```python
from build123d import *

# Parameters (mm, degrees)
EXTRUDE_275_DEPTH = 17
SKETCH_2_R        = 12.9
EXTRUDE_1_DEPTH   = 200
FILLET_3_R        = 2
SKETCH_3_R        = 11
EXTRUDE_2_DEPTH   = 100
FILLET_4_R        = 2


with BuildPart() as part:
    # 草图1 → Extrude 275 (new body)
    with BuildSketch(Plane.XY):
        Polygon((20.984201837, 10.954296262), (1.005402075, 23.65), (-19.978799762, 12.695703738), (-20.984201837, -10.954296262), (-1.005402075, -23.65), (19.978799762, -12.695703738), align=None)
    extrude(amount=EXTRUDE_275_DEPTH)

    # 草图2 → 凸台-拉伸1 (add)
    with BuildSketch(Plane.XY.offset(17)):
        with Locations(Location((0, 0, 0), (0, 0, 180))):
            Circle(SKETCH_2_R)
    extrude(amount=EXTRUDE_1_DEPTH)

    # 圆角3
    fillet_3_edges = [part.edges().sort_by_distance(p)[0] for p in [
        (9.486698843, -18.172851869, 0),
        (-10.994801956, -17.302148131, 0),
        (-20.4815008, 0.870703738, 0),
        (-9.486698843, 18.172851869, 0),
        (10.994801956, 17.302148131, 0),
        (20.4815008, -0.870703738, 0),
    ]]
    fillet(fillet_3_edges, radius=FILLET_3_R)

    # 草图3 → 凸台-拉伸2 (add)
    with BuildSketch(Plane.XY.offset(217)):
        Circle(SKETCH_3_R)
    extrude(amount=EXTRUDE_2_DEPTH)

    # 圆角4
    fillet_4_edges = [part.edges().sort_by_distance(p)[0] for p in [
        (-11, 0, 317),
    ]]
    fillet(fillet_4_edges, radius=FILLET_4_R)


solid = part.part
```
Source: CAD feature listing. Evaluate the final solid. Frame: model axes, mm. A direction names the side the tool comes from. Coordinates: 2 decimals unless noted, no trailing zeros. Order: outer loops, then holes, each group sorted by start corner. A loop starts at its lowest first (then second) coordinate and runs counter-clockwise, first axis right, second up. Notation, with made-up numbers: M 2.25,51 L 58.25,51 A34 cw 58.25,83 Z; hole C 89,-32 d6. An arc over 180 degrees is marked long. Write each question's results on one line, items separated by ' | '. Start each with the question number.
1) Access query for faces 1 (the face through (-11.135, -17.213, 9.395)), 2 (the face through (9, -10, 17)). Directions: +Z, -Z, +X, -X, +Y, -Y. A direction counts if a zero-diameter tool reaches every point of the face in a straight line with its end or side. Return the directions, or none.
2) Section query A-A (z = 85). Return the cut outline in (x, y).
3) Line query: line 1 (X direction, y = 2, z = 62); line 2 (Z direction, x = -16.5, y = 12); line 3 (Y direction, x = -1, z = 29.5). Output: solid intervals per line, ascending. Write a range as from..to.
4) Contact query for flat-ended pins moving along their axis: pin 1 Ø10 at (x, z) = (-3.5, 179.5) entering from -Y; pin 2 Ø12 at (x, y) = (9, -13.5) entering from +Z; pin 3 Ø1.5 at (y, z) = (-11.5, 154.5) entering from +X. Output: stop coordinate, or through.
Answers:
1) face 1: +Z, -Z, -X, -Y | face 2: +Z
2) outline: C 0,0 d25.8
3) line 1: x = -12.74..12.74 | line 2: z = 0..17 | line 3: y = -12.86..12.86
4) pin 1: stops at y = -12.9 | pin 2: stops at z = 316.58 | pin 3: stops at x = 7.13
